Geometry check sheet. Reference: the model listing, model coordinates, mm. A direction names the side the tool comes from. Give positions to 0.01 mm unless a question says otherwise; leave off trailing zeros. Write each loop counter-clockwise with the first axis right and the second up, starting at its lowest first coordinate (ties: lowest second). Pieces come first, ordered by that corner, then holes. Notation, with made-up numbers: (50.25, 52.5) - (65.25, 52.5) arc R21 cw to (65.25, 74.5) - close; hole circle Ø4 at (1, 30.5). An arc over 180 degrees is marked (long way). Write item = value, one per line. Start each with the question number.
(1) Access from +Z, -Z, +X, -X, +Y, -Y to the whole of each face (thin tool, end or side, straight path). Record for faces 1 (the cylindrical face through (6.691, -12.864, 61.975)), 2 (the cylindrical face through (-13.887, -10.648, 12.325)).
(2) Depth check by flat-ended pin: pin 1 Ø4 at (x, z) = (0.5, 60.5) entering from -Y; pin 2 Ø6 at (y, z) = (-8, 151) entering from +X; pin 3 Ø2 at (x, z) = (2.5, 120.5) entering from +Y. Enter the tip coordinate at first touch or a pass-through.
(3) Section check A-A, the plane y = 0. Enter the section's corners in (x, z), plus the area to 4 significant figures.
(4) Section check C-C, the plane z = 124.5. Enter the section's corners in (x, y), plus the area to 3 significant figures.
(5) Thickness scan on L1, parallel to Y at x = -1, z = 75.5; L2, parallel to Z at x = -3, y = -16; L3, parallel to Z at x = 11.5, y = -8.5. Record the ranges inside material, lowest first.
```python
from build123d import *

# Parameters (mm, degrees)
F0_R     = 13.5
F1_DEPTH = 195
F2_R     = 17.5
F3_DEPTH = 25
F4_R     = 14.5
F5_DEPTH = 100


with BuildPart() as f1:
    # F0 (on Top) → F1 (new body)
    with BuildSketch(Plane.XY):
        Circle(F0_R)
    extrude(amount=F1_DEPTH)

    # F2 (on Top) → F3 (join)
    with BuildSketch(Plane.XY):
        Circle(F2_R)
    extrude(amount=F3_DEPTH)

    # F4 (on Top) → F5 (join)
    with BuildSketch(Plane.XY):
        Circle(F4_R)
    extrude(amount=F5_DEPTH)


solid = f1.part
```
Model answer:
q1.face_1 = +Z
q1.face_2 = +Z, -Z
q2.pin_1 = -14.5
q2.pin_2 = 12.54
q2.pin_3 = 13.42
q3.outline = (-17.5, 0) - (17.5, 0) - (17.5, 25) - (14.5, 25) - (14.5, 100) - (13.5, 100) - (13.5, 195) - (-13.5, 195) - (-13.5, 100) - (-14.5, 100) - (-14.5, 25) - (-17.5, 25) - close
q3.area = 5,615 mm²
q4.outline = circle Ø27 at (0, 0)
q4.area = 573 mm²
q5.L1 = -14.47 to 14.47
q5.L2 = 0 to 25
q5.L3 = 0 to 100
